Autodesk Inventor part; units mm, degrees
ref_plane "YZ Plane" through (0, 0, 0) normal (1, 0, 0) x (0, 1, 0)
ref_plane "XZ Plane" through (0, 0, 0) normal (0, 1, 0) x (-1, 0, 0)
ref_plane "XY Plane" through (0, 0, 0) normal (0, 0, 1) x (1, 0, 0)
sketch "Sketch1" plane through (0, 0, 0) normal (0, 0, 1) x (1, 0, 0)
  line L0 (0, 0) -> (25.4, 0)
  line L1 (25.4, 0) -> (25.4, 3.175)
  line L2 (3.175, 50.8) -> (0, 50.8)
  line L3 (0, 50.8) -> (0, 0)
  line L4 (3.175, 50.8) -> (3.175, 3.175)
  line L5 (3.175, 3.175) -> (25.4, 3.175)
  dimension "d0" = 50.8
  dimension "d1" = 25.4
  dimension "d2" = 3.175
  dimension "d3" = 3.175
extrude "Extrusion1" add sketch "Sketch1" along normal blind 203.2
sketch "Sketch2" plane through (0, 0, 0) normal (-1, 0, 0) x (0, 0, 1)
  line L0 (203.2, 0) -> (203.2, 50.8)
  line L1 (0, 50.8) -> (203.2, 50.8)
  circle A0 centre (123.19, 25.4) radius 14.2875
  circle A1 centre (161.29, 25.4) radius 14.2875
  dimension "d6" = 28.575
  dimension "d7" = 28.575
  dimension "d8" = 25.4
  dimension "d9" = 41.91
  dimension "d10" = 38.1
extrude "Extrusion2" cut sketch "Sketch2" against normal blind 203.2
equation "\"d6\" = d7"
properties part number "manipulator bearing back right"
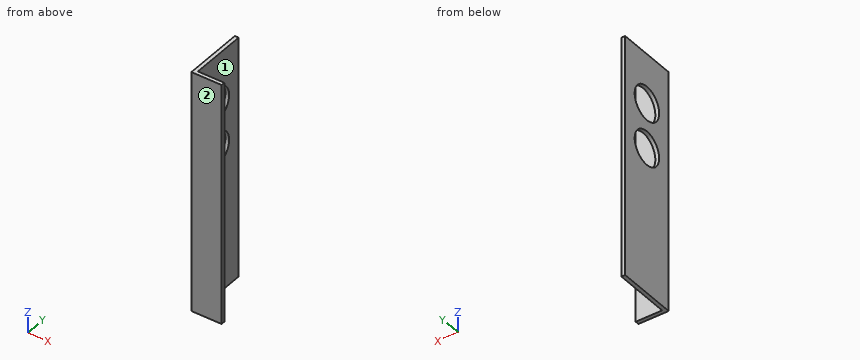
Could you check a few things on this model? Use its own coordinates, in mm. Face numbers are marked on the shaded views. A direction names the side the tool comes from. Coordinates: 2 decimals unless noted, no trailing zeros. Write each loop counter-clockwise with the first axis right and the second up, starting at its lowest first coordinate (ties: lowest second). Pieces come first, ordered by that corner, then holes. Notation, with made-up numbers: (68, 57.25) -> (74, 57.25) arc R13 ccw to (74, 72.25) -> close; hole circle Ø11 at (7, 47). An arc over 180 degrees is marked (long way). Write item = value, one per line. Start each with the question number.
(1) Will these pins go through, and if not, where does the flat tip stop? pin 1 (10 mm diameter, centred on y = 13, z = 162.5, fed in from +X) (3 decimals); pin 2 (5 mm diameter, centred on x = 9, z = 111.5, fed in from +Y) (3 decimals).
(2) I want a section at C-C (x = 16.5). Please give me the cut outline in (y, z) (3 decimals).
(3) Which directions (+Z, -Z, +X, -X, +Y, -Y) give clear straight access to the entire face, cutting with the end or side of a thin tool? Please do the marked faces 1 and 2.
(4) I want a section at A-A (y = 25.4). Please give me the cut outline in (x, z) (1 decimal).
(5) I want a section at B-B (z = 161.29). Please give me the cut outline in (x, y) (1 decimal).
(6) I need wall thicknesses on line 1 (Y direction, x = 1.25, z = 161.29); line 2 (X direction, y = 7, z = 116) (3 decimals). Which ranges of each line are inside material? Lowest first, please. Write a range as [from, to].
Result set:
q1.pin_1 = 3.175
q1.pin_2 = 3.175
q2.outline = (0, 0) -> (3.175, 0) -> (3.175, 203.2) -> (0, 203.2) -> close
q3.face_1 = +Z, -Z, +X, +Y
q3.face_2 = +Z, -Z, +X, -X, -Y
q4.outline = (0, 0) -> (3.2, 0) -> (3.2, 108.9) -> (0, 108.9) -> close; (0, 137.5) -> (3.2, 137.5) -> (3.2, 147) -> (0, 147) -> close; (0, 175.6) -> (3.2, 175.6) -> (3.2, 203.2) -> (0, 203.2) -> close
q5.outline = (0, 0) -> (25.4, 0) -> (25.4, 3.2) -> (3.2, 3.2) -> (3.2, 11.1) -> (0, 11.1) -> close; (0, 39.7) -> (3.2, 39.7) -> (3.2, 50.8) -> (0, 50.8) -> close
q6.line_1 = [0, 11.11], [39.69, 50.8]
q6.line_2 = [0, 3.175]
